Input: part model. Units: mm. Frame: model coordinates. A direction names the side the tool comes from. Round coordinates to 2 decimals unless told otherwise and drop trailing zeros. Write each loop counter-clockwise with the first axis right and the second up, starting at its lowest first coordinate (ties: lowest second). Pieces come first, ordered by that corner, then holes. Notation, with made-up numbers: (60, 75.25) - (113, 75.25) arc R20 ccw to (113, 83.25) - close; hole circle Ø11 at (51, 54). An arc over 180 degrees is marked (long way). Use one line per item in the form item = value.
```python
from build123d import *

# Parameters (mm, degrees)
SKETCH_1_R       = 1.25
BOARD_DEPTH      = 1
SKETCH_2_W       = 38
SKETCH_2_H       = 30
SCREEN_DEPTH     = 2
SCREEN_RADIUS_R  = 3.5
SKETCH_3_W       = 51
SKETCH_3_H       = 5
PLUG_DEPTH       = 7.5
SKETCH_4_W       = 15.14
SKETCH_4_H       = 20
SPEAKER_DEPTH    = 5
SKETCH_5_W       = 4.5
SKETCH_5_H       = 2.5
BUTTON_DEPTH     = 3.4
SKETCH_6_R       = 1
BUTTON_TAP_DEPTH = 1
SKETCH_7_W       = 1.5
SKETCH_7_H       = 1.5
RGB_LED_DEPTH    = 0.7
SKETCH_8_W       = 3.2
SKETCH_8_H       = 2.5
MIC_DEPTH        = 1.3
EXTRUDE_START    = 0.1
EXTRUDE_1_DEPTH  = 0.1


with BuildPart() as part:
    # 草图1 → board (new body)
    with BuildSketch(Plane(origin=(0, 0, 0), x_dir=(1, 0, 0), z_dir=(0, 1, 0))):
        with BuildLine():
            Line((-29.5, 15), (29.5, 15))
            ThreePointArc((29.5, 15), (31.621320344, 14.121320344), (32.5, 12))
            Line((32.5, 12), (32.5, -12))
            ThreePointArc((32.5, -12), (31.621320344, -14.121320344), (29.5, -15))
            Line((29.5, -15), (-29.5, -15))
            ThreePointArc((-29.5, -15), (-31.621320344, -14.121320344), (-32.5, -12))
            Line((-32.5, -12), (-32.5, 12))
            ThreePointArc((-32.5, 12), (-31.621320344, 14.121320344), (-29.5, 15))
        make_face()
        with Locations(Location((-29.5, 12, 0), (0, 0, 270))):
            Circle(SKETCH_1_R, mode=Mode.SUBTRACT)
        with Locations(Location((29.5, 12, 0), (0, 0, 270))):
            Circle(SKETCH_1_R, mode=Mode.SUBTRACT)
        with Locations(Location((-29.5, -12, 0), (0, 0, 270))):
            Circle(SKETCH_1_R, mode=Mode.SUBTRACT)
        with Locations(Location((29.5, -12, 0), (0, 0, 270))):
            Circle(SKETCH_1_R, mode=Mode.SUBTRACT)
    extrude(amount=BOARD_DEPTH)

    # 草图2 → screen (add)
    with BuildSketch(Plane(origin=(0, 1, 0), x_dir=(1, 0, 0), z_dir=(0, 1, 0))):
        with Locations((7.5, 0)):
            Rectangle(SKETCH_2_W, SKETCH_2_H)
    extrude(amount=SCREEN_DEPTH)

    # screen-radius
    screen_radius_edges = [part.edges().sort_by_distance(p)[0] for p in [
        (-11.5, 2, -15),
        (-11.5, 2, 15),
        (26.5, 2, 15),
        (26.5, 2, -15),
    ]]
    fillet(screen_radius_edges, radius=SCREEN_RADIUS_R)

    # 草图3 → plug (add)
    with BuildSketch(Plane.XZ):
        with Locations((0, -11.5)):
            Rectangle(SKETCH_3_W, SKETCH_3_H)
    extrude(amount=PLUG_DEPTH)

    # 草图4 → speaker (add)
    with BuildSketch(Plane.XZ):
        with Locations((-17.52, 2.68)):
            Rectangle(SKETCH_4_W, SKETCH_4_H)
    extrude(amount=SPEAKER_DEPTH)

    # 草图5 → button (add)
    with BuildSketch(Plane.XZ):
        with Locations((5.65, 13.25)):
            Rectangle(SKETCH_5_W, SKETCH_5_H)
    extrude(amount=BUTTON_DEPTH)

    # 草图6 → button-tap (add)
    with BuildSketch(Plane.XY.offset(14.5)):
        with Locations(Location((5.65, -1.7, 0), (0, 0, 180))):
            Circle(SKETCH_6_R)
    extrude(amount=BUTTON_TAP_DEPTH)

    # 草图7 → rgb-led (add)
    with BuildSketch(Plane(origin=(0, 1, 0), x_dir=(1, 0, 0), z_dir=(0, 1, 0))):
        with Locations((29.25, 0)):
            Rectangle(SKETCH_7_W, SKETCH_7_H)
    extrude(amount=RGB_LED_DEPTH)

    # 草图8 → mic (add)
    with BuildSketch(Plane(origin=(0, 1, 0), x_dir=(1, 0, 0), z_dir=(0, 1, 0))):
        with Locations((-26.6, -0.25)):
            Rectangle(SKETCH_8_W, SKETCH_8_H)
    extrude(amount=MIC_DEPTH)

    # 草图9 → 凸台-拉伸1 (add)
    with BuildSketch(Plane(origin=(0, 3, 0), x_dir=(1, 0, 0), z_dir=(0, 1, 0)).offset(EXTRUDE_START)):
        with BuildLine():
            Line((26.5, -11.5), (26.5, 11.5))
            ThreePointArc((26.5, 11.5), (25.80624304, 13.591650066), (24, 14.854101966))
            Line((24, 14.854101966), (24, -14.854101966))
            ThreePointArc((24, -14.854101966), (25.80624304, -13.591650066), (26.5, -11.5))
        make_face()
    extrude(amount=-EXTRUDE_1_DEPTH)


solid = part.part
```
(1) First-contact query: pin 1 Ø12 at (x, z) = (-14.5, 4) entering from +Y; pin 2 Ø4 at (y, z) = (-3, 2.5) entering from +X; pin 3 Ø4 at (x, z) = (-29.5, -12) entering from +Y. Flat tips, straight axial feed; report the tip coordinate or a pass-through.
Derived:
pin_1 = 3
pin_2 = -9.95
pin_3 = 1
(2) Cut plane B-B on x = 10. Output: boundary loops of the cut face in (y, z), then the cut area to 4 significant figures.
Derived:
outline = (-7.5, -14) - (0, -14) - (0, -15) - (3, -15) - (3, 15) - (0, 15) - (0, -9) - (-7.5, -9) - close
area = 127.5 mm^2
(3) Access query for faces 4 (the face through (-25.5, -4, -12)), 5 (the face through (29, 1.7, 0)), 6 (the face through (-18, -2, 12.68)), 7 (the face through (-27, 2, 1.5)). Directions: +Z, -Z, +X, -X, +Y, -Y. A direction counts if a zero-diameter tool reaches every point of the face in a straight line with its end or side. Return the directions, or none.
Derived:
face_4 = +Z, -Z, -X, -Y
face_5 = +Z, -Z, +X, +Y
face_6 = +Z, -X, -Y
face_7 = +Z, -X, +Y
(4) Cut plane A-A on y = -1.7. Output: boundary loops of the cut face in (x, z).
Derived:
outline = (-25.5, -14) - (25.5, -14) - (25.5, -9) - (-25.5, -9) - close; (-25.09, -7.32) - (-9.95, -7.32) - (-9.95, 12.68) - (-25.09, 12.68) - close; (3.4, 12) - (7.9, 12) - (7.9, 14.5) - (6.65, 14.5) - (6.65, 15.5) - (4.65, 15.5) - (4.65, 14.5) - (3.4, 14.5) - close
(5) Cut plane D-D on y = -5.75. Output: boundary loops of the cut face in (x, z), then the cut area to 3 significant figures.
Derived:
outline = (-25.5, -14) - (25.5, -14) - (25.5, -9) - (-25.5, -9) - close
area = 255 mm^2
(6) Cut plane C-C on z = 4.5. Output: boundary loops of the cut face in (x, y), then the cut area to 3 significant figures.
Derived:
outline = (-32.5, 0) - (-25.09, 0) - (-25.09, -5) - (-9.95, -5) - (-9.95, 0) - (32.5, 0) - (32.5, 1) - (26.5, 1) - (26.5, 3.1) - (24, 3.1) - (24, 3) - (-11.5, 3) - (-11.5, 1) - (-32.5, 1) - close
area = 217 mm^2
(7) Draft query along Z for faces 1 (the face through (-25.09, -2, 3)), 2 (the face through (-27, 2, -1)), 3 (the face through (-18, -2, -7.32)). Return one class per face: released by +Z, released by -Z, zero draft, split by the parting line, or undercut.
Derived:
face_1 = zero draft
face_2 = released by -Z
face_3 = undercut
(8) Material intervals for L1, parallel to X at y = 0.35, z = 12; L2, parallel to Z at x = -11.5, y = -2; L3, parallel to Y at x = 4, z = 7, sorted ascending.
Derived:
L1 = -32.5 to -30.75, -28.25 to 28.25, 30.75 to 32.5
L2 = -14 to -9, -7.32 to 12.68
L3 = 0 to 3
